The model under review builds one solid part; all positions refer to its coordinate system, in mm. A direction names the side the tool comes from. Coordinates: 2 decimals unless noted, no trailing zeros. Loops run counter-clockwise (first coordinate to the right, second up) from the corner with the lowest first, then second, coordinate; pieces in that order, holes last. Notation, with made-up numbers: (43, 35.5) -> (67, 35.5) arc R13 ccw to (67, 50.5) -> close; hole circle Ø6 at (-33, 57.5). An arc over 180 degrees is marked (long way). One line per question, with ' | ' between items. Start each with the question number.
from build123d import *

# Parameters (mm, degrees)
SKETCH1_R           = 1.5
BOSS_EXTRUDE1_DEPTH = 5
CUT_EXTRUDE2_DEPTH  = 6


with BuildPart() as part:
    # Sketch1 → Boss-Extrude1 (new body)
    with BuildSketch(Plane.XY):
        Polygon((-13.5, 0), (13.5, 0), (13.5, 24), (18.5, 24), (18.5, 49), (13.5, 49), (13.5, 64), (-13.5, 64), (-13.5, 49), (-18.5, 49), (-18.5, 24), (-13.5, 24), align=None)
        with Locations((0, 43.75)):
            Circle(SKETCH1_R, mode=Mode.SUBTRACT)
    extrude(amount=BOSS_EXTRUDE1_DEPTH)

    # Sketch2 → Cut-Extrude2 (cut, through all)
    with BuildSketch(Plane.XY.offset(5)):
        Polygon((-13.5, 56.5), (-13.5, 57.7), (-9.5, 57.7), (-9.5, 59.25), (-7.7, 59.25), (-7.7, 57.654169795), (-5.7, 57.654169795), (-5.7, 55.345830205), (-7.7, 55.345830205), (-7.7, 53.75), (-9.5, 53.75), (-9.5, 55.3), (-13.5, 55.3), align=None)
        Polygon((13.5, 56.5), (13.5, 55.3), (9.5, 55.3), (9.5, 53.75), (7.7, 53.75), (7.7, 55.345830205), (5.7, 55.345830205), (5.7, 57.654169795), (7.7, 57.654169795), (7.7, 59.25), (9.5, 59.25), (9.5, 57.7), (13.5, 57.7), align=None)
        Polygon((-13.5, 10.8), (-13.5, 13.2), (-9.5, 13.2), (-9.5, 14.75), (-7.7, 14.75), (-7.7, 13.2), (-5.7, 13.2), (-5.7, 10.8), (-7.7, 10.8), (-7.7, 9.25), (-9.5, 9.25), (-9.5, 10.8), align=None)
        Polygon((13.5, 10.8), (9.5, 10.8), (9.5, 9.25), (7.7, 9.25), (7.7, 10.8), (5.7, 10.8), (5.7, 13.2), (7.7, 13.2), (7.7, 14.75), (9.5, 14.75), (9.5, 13.2), (13.5, 13.2), align=None)
    extrude(amount=-CUT_EXTRUDE2_DEPTH, mode=Mode.SUBTRACT)


solid = part.part
1) Consider section D-D, the plane y = 57. Write out the cut boundary in (x, z), plus the area to 3 significant figures.
2) Wall thickness on L1, parallel to Y at x = -12, z = 2.95; L2, parallel to X at y = 9.5, z = 0.95; L3, parallel to Y at x = 9, z = 0.8: over which ranges is each line inside the solid? List them lowest first.
3) Machinability: for faces 1 (the face through (-7.7, 55, 3)), 2 (the face through (13.5, 52, 2)), 3 (the face through (-7, 10.8, 3)), which of the approach directions +Z, -Z, +X, -X, +Y, -Y give a long, thin tool a straight path to every point of the face, cutting with its end or side? Answer none if there is none.
4) Insertion check: pin 1 Ø2.5 at (y, z) = (12, 2) entering from -X; pin 2 Ø4 at (x, y) = (6, 12) entering from -Z; pin 3 Ø1.7 at (y, z) = (58, 2) entering from +X; pin 4 Ø1.2 at (y, z) = (12, 2) entering from +X. Each pin has a flat end and moves straight along its axis. Give the tip position at first contact, or say it passes through.
5) Consider section C-C, the plane y = 43.75. Write out the cut boundary in (x, z), plus the area to 3 significant figures.
6) Consider section A-A, the plane x = 12. Write out the cut boundary in (y, z).
7) Consider section B-B, the plane x = 0. Write out the cut boundary in (y, z).
8) Mouldability with a two-part tool opening along Y and no side actions: class faces 4 (the face through (7, 57.654, 3)), 5 (the face through (0, 64, 2)), 6 (the face through (13.5, 61, 2)) as +Y half, -Y half, draft (parallel to the pull), parting line (faces both ways), or undercut.
Filled sheet:
1) outline: (-5.7, 0) -> (5.7, 0) -> (5.7, 5) -> (-5.7, 5) -> close | area: 57.0 mm^2
2) L1: 0 to 10.8, 13.2 to 55.3, 57.7 to 64 | L2: -13.5 to -9.5, -7.7 to 7.7, 9.5 to 13.5 | L3: 0 to 9.25, 14.75 to 53.75, 59.25 to 64
3) face 1: +Z, -Z | face 2: +Z, -Z, +X, +Y | face 3: +Z, -Z, -X
4) pin 1: x = -13.5 | pin 2: z = 0 | pin 3: x = 13.5 | pin 4: x = 5.7
5) outline: (-18.5, 0) -> (-1.5, 0) -> (-1.5, 5) -> (-18.5, 5) -> close; (1.5, 0) -> (18.5, 0) -> (18.5, 5) -> (1.5, 5) -> close | area: 170 mm^2
6) outline: (0, 0) -> (10.8, 0) -> (10.8, 5) -> (0, 5) -> close; (13.2, 0) -> (55.3, 0) -> (55.3, 5) -> (13.2, 5) -> close; (57.7, 0) -> (64, 0) -> (64, 5) -> (57.7, 5) -> close
7) outline: (0, 0) -> (42.25, 0) -> (42.25, 5) -> (0, 5) -> close; (45.25, 0) -> (64, 0) -> (64, 5) -> (45.25, 5) -> close
8) face 4: undercut | face 5: +Y half | face 6: draft
